from build123d import *

# Parameters (mm, degrees)
F1_W     = 77.435985
F1_H     = 77.229559
F1_R     = 26.671877
F2_DEPTH = 10


with BuildPart() as f2:
    # F1 (on face) → F2 (new body)
    with BuildSketch(Plane.XZ):
        with Locations((-38.717993, -38.614779)):
            Rectangle(F1_W, F1_H)
        with Locations((-39.945371, -36.837861)):
            Circle(F1_R, mode=Mode.SUBTRACT)
    extrude(amount=F2_DEPTH)


solid = f2.part
The model under review builds one solid part; all positions refer to its coordinate system, in mm. Round coordinates to 2 decimals unless told otherwise and drop trailing zeros. Loops run counter-clockwise (first coordinate to the right, second up) from the corner with the lowest first, then second, coordinate; pieces in that order, holes last. Notation, with made-up numbers: (-18, 86) -> (24, 86) arc R29 cw to (24, 120) -> close; hole circle Ø2 at (26.25, 11). An arc over 180 degrees is marked (long way). Answer as CSV lines item,"result".
1) Add section A-A on x = -42. Write out the cut boundary in (y, z), plus the area to 3 significant figures.
Geometry results:
outline,"(-10, -77.23) -> (0, -77.23) -> (0, -63.43) -> (-10, -63.43) -> close; (-10, -10.25) -> (0, -10.25) -> (0, 0) -> (-10, 0) -> close"
area,"240 mm²"
2) Draft analysis for pull direction X (two halves, no side actions). For faces 1 (the face through (-39, -5, 0)), 2 (the face through (-61.11, -4.93, -53.07)), 3 (the face through (0, -5, -39)), state which applies: pulls with the +X half, pulls with the -X half, needs draft (parallel to the pull), parting line crosses it, or undercut.
Geometry results:
face 1,"needs draft"
face 2,"undercut"
face 3,"pulls with the +X half"
3) Add section B-B on z = -42. Write out the cut boundary in (x, y).
Geometry results:
outline,"(-77.44, -10) -> (-66.11, -10) -> (-66.11, 0) -> (-77.44, 0) -> close; (-13.78, -10) -> (0, -10) -> (0, 0) -> (-13.78, 0) -> close"
4) Add section C-C on y = -3.5. Write out the cut boundary in (x, z), plus the area to 3 significant figures.
Geometry results:
outline,"(-77.44, -77.23) -> (0, -77.23) -> (0, 0) -> (-77.44, 0) -> close; hole circle Ø53.34 at (-39.95, -36.84)"
area,"3,750 mm²"
5) To check wall thickness, follow line 1 along Z through (x, y) = (-32, -4.25); line 2 along Z through (x, y) = (-25, -6.5); line 3 along X through (y, z) = (-4, -55.5). State the ranges of each line that lie inside material, in increasing order. Write a range as from..to.
Geometry results:
line 1,"z = -77.23..-62.3, -11.38..0"
line 2,"z = -77.23..-58.93, -14.75..0"
line 3,"x = -77.44..-59, -20.89..0"
